from build123d import *

# Parameters (mm, degrees)
BOSS_EXTRUDE1_DEPTH = 20.32
SKETCH2_W           = 24.5618
SKETCH2_H           = 13.97
CUT_EXTRUDE1_DEPTH  = 24.5618
CUT_EXTRUDE2_DEPTH  = 43.389008236
CIRPATTERN1_COUNT   = 2
CIRPATTERN1_ANGLE   = 270


with BuildPart() as part:
    # Sketch1 → Boss-Extrude1 (new body)
    with BuildSketch(Plane.XY):
        Polygon((0, 0), (0, 27.94), (5.842, 27.94), (5.842, 23.495), (23.495, 5.842), (27.94, 5.842), (27.94, 0), align=None)
    extrude(amount=-BOSS_EXTRUDE1_DEPTH)

    # Sketch2 → Cut-Extrude1 (cut)
    with BuildSketch(Plane(origin=(0, 27.94, 0), x_dir=(1, 0, 0), z_dir=(0, 1, 0))):
        with Locations((15.6591, 10.16)):
            Rectangle(SKETCH2_W, SKETCH2_H)
    extrude(amount=-CUT_EXTRUDE1_DEPTH, mode=Mode.SUBTRACT)

    # Sketch3 → Cut-Extrude2 (cut, through all)
    with BuildSketch(Plane(origin=(0, 3.3782, 0), x_dir=(1, 0, 0), z_dir=(0, 1, 0))):
        with BuildLine():
            Line((13.462, 13.462), (17.018, 13.462))
            ThreePointArc((17.018, 13.462), (20.32, 10.16), (17.018, 6.858))
            Line((17.018, 6.858), (13.462, 6.858))
            ThreePointArc((13.462, 6.858), (10.16, 10.16), (13.462, 13.462))
        make_face()
    cut_extrude2 = extrude(amount=-CUT_EXTRUDE2_DEPTH, mode=Mode.SUBTRACT)

    # CirPattern1: Cut-Extrude2 ×2 about axis
    cirpattern1_axis = Axis((0, 0, -20.32), (0, 0, -1))
    for i in range(1, CIRPATTERN1_COUNT):
        add(cut_extrude2.rotate(cirpattern1_axis, i * CIRPATTERN1_ANGLE / (CIRPATTERN1_COUNT - 1)), mode=Mode.SUBTRACT)


solid = part.part
Geometry check sheet. Reference: the model listing, model coordinates, mm. A direction names the side the tool comes from. Give positions to 0.01 mm unless a question says otherwise; leave off trailing zeros. Loops run counter-clockwise (first coordinate to the right, second up) from the corner with the lowest first, then second, coordinate; pieces in that order, holes last. Notation, with made-up numbers: M -12.5,57 L 12.5,57 A14 ccw 12.5,84 Z; hole C 64,70.5 d4. An arc over 180 degrees is marked long. Write each question's results on one line, items separated by ' | '.
1) Tool access check on faces 4 (the face through (3.378, 19, -13)), 5 (the face through (10.16, 1.71, -10.09)), 6 (the face through (5.842, 26, -19)). Record the directions out of +Z, -Z, +X, -X, +Y, -Y that give a thin tool (end or side, any length) a straight path to the whole face; none if there is none.
Answers follow:
face 4: +X, +Y | face 5: +Y, -Y | face 6: +Z, -Z, +X, +Y
2) Section check A-A, the plane z = -10.16. Record the boundary of the cut face in (x, y), plus the area to 3 significant figures.
Answers follow:
outline: M 0,0 L 10.16,0 L 10.16,3.38 L 3.38,3.38 L 3.38,10.16 L 0,10.16 Z; M 0,20.32 L 3.38,20.32 L 3.38,27.94 L 0,27.94 Z; M 20.32,0 L 27.94,0 L 27.94,3.38 L 20.32,3.38 Z | area: 109 mm2
3) Section check C-C, the plane x = 17.5. Record the boundary of the cut face in (y, z) (3 decimals), plus the area to 3 significant figures.
Answers follow:
outline: M 0,-20.32 L 11.837,-20.32 L 11.837,-17.145 L 3.378,-17.145 L 3.378,-13.427 L 0,-13.427 Z; M 0,-6.893 L 3.378,-6.893 L 3.378,-3.175 L 11.837,-3.175 L 11.837,0 L 0,0 Z | area: 100 mm2
4) Section check D-D, the plane z = -6.25. Record the boundary of the cut face in (x, y), plus the area to 3 significant figures.
Answers follow:
outline: M 0,0 L 27.94,0 L 27.94,3.38 L 3.38,3.38 L 3.38,27.94 L 0,27.94 Z | area: 177 mm2
5) Section check B-B, the plane y = 2.5. Record the boundary of the cut face in (x, z).
Answers follow:
outline: M 0,-20.32 L 27.94,-20.32 L 27.94,0 L 0,0 Z; hole M 13.46,-13.46 L 17.02,-13.46 A3.3 ccw 17.02,-6.86 L 13.46,-6.86 A3.3 ccw Z
6) Gauge pin test, flat ends, axial feed: pin 1 (1 mm diameter, centred on y = 25.5, z = -19, fed in from +X); pin 2 (1 mm diameter, centred on x = 25.5, z = -1.5, fed in from +Y); pin 3 (4 mm diameter, centred on x = 12, z = -13.5, fed in from +Y); pin 4 (6 mm diameter, centred on x = 17.5, y = 17.5, fed in from -Z). Record the tip position at first contact, or that the pin passes through.
Answers follow:
pin 1: x = 5.84 | pin 2: y = 5.84 | pin 3: y = 3.38 | pin 4: through
7) Thickness scan on line 1 (Z direction, x = 12.25, y = 13.75) (3 decimals); line 2 (Z direction, x = 17, y = 3.25); line 3 (X direction, y = 26.25, z = -18.25). Record the ranges inside material, lowest first.
Answers follow:
line 1: -20.32 to -17.145, -3.175 to 0 | line 2: -20.32 to -13.46, -6.86 to 0 | line 3: 0 to 5.84
8) Release check for a two-part mould opening along Y. For faces 1 (the face through (2, 15, -6.858)), 2 (the face through (15, 2, -6.858)), 3 (the face through (15, 3.378, -15)) record: +Y half, -Y half, draft (parallel to the pull), parting line (faces both ways), or undercut.
Answers follow:
face 1: undercut | face 2: draft | face 3: +Y half
